Read the model definition and answer for the solid it produces. Units are mm, in the model's axes. A direction names the side the tool comes from. Coordinates: 2 decimals unless noted, no trailing zeros. Loops run counter-clockwise (first coordinate to the right, second up) from the corner with the lowest first, then second, coordinate; pieces in that order, holes last. Notation, with made-up numbers: M -32,-8.75 L 16,-8.75 A20 ccw 16,15.25 Z; hole C 81.25,58.25 d5. An arc over 180 degrees is marked long. One line per item, written item: value. Start each with the question number.
1. Consider probe 1 along Z at (x, y) = (-10, -9.3); probe 2 along Z at (x, y) = (17, 0.25); probe 3 along Y at (x, z) = (26.5, 3.5). Determine where each line is inside the solid, lowest interval first.
2. Flat-ended cylindrical pins translate along their axes: pin 1 (2.5 mm diameter, centred on x = 13, y = 2.5, fed in from +Z); pin 2 (2 mm diameter, centred on y = -2.5, z = 19, fed in from -X); pin 3 (4 mm diameter, centred on y = -5.5, z = 48, fed in from +X). Find the tip coordinate at first contact, or state that the pin passes through.
3. The part is cut by section C-C (y = -8.5). Write down the section's boundary in (x, z).
4. The part is cut by section A-A (x = -10). Write down the section's boundary in (y, z).
5. Determine the mould class of faces 4 (the face through (0, -1, 30)), 5 (the face through (19, -1.95, 4)), 6 (the face through (4, -4.1, 23)) for opening direction Y: +Y half, -Y half, draft (parallel to the pull), parting line (faces both ways), or undercut.
6. For faces 1 (the face through (5.039, -1, 56)), 2 (the face through (-12, -7.081, 3)), 3 (the face through (7, 1, 55)), determine the directions among +Z, -Z, +X, -X, +Y, -Y from which every point of the face is accessible in a straight line to the end or side of a thin tool.
```python
from build123d import *

# Parameters (mm, degrees)
PAD_DEPTH       = 12
SKETCH001_R     = 3
HOLE_DEPTH      = 13.001
PAD001_DEPTH    = 7
SKETCH003_W     = 28
SKETCH003_H     = 2.7
POCKET_DEPTH    = 2
SKETCH004_W     = 4
SKETCH004_H     = 2.7
POCKET001_DEPTH = 2.5


with BuildPart() as part:
    # Sketch → Pad (new body)
    with BuildSketch(Plane.XY):
        Polygon((-20, -10.081048), (5, -10.081048), (5, 2.918952), (0, 2.918952), (0, -7.081048), (-20, -7.081048), align=None)
    extrude(amount=PAD_DEPTH)

    # Sketch001 (on Face1 of Pad) → Hole (cut, through all)
    with BuildSketch(Plane.XZ.offset(10.081048)):
        with Locations((-10, 6)):
            Circle(SKETCH001_R)
    extrude(amount=-HOLE_DEPTH, mode=Mode.SUBTRACT)

    # Sketch002 → Pad001 (join)
    with BuildSketch(Plane.XZ.offset(-2.9)):
        Polygon((33.008904, 5), (33.008904, 0), (0, 0), (0, 11.991246), (0, 60), (9.008904, 60), (9.008904, 55), (5.008904, 55), (5.008904, 5), align=None)
    extrude(amount=PAD001_DEPTH)

    # Sketch003 (on Face15 of Pad001) → Pocket (cut)
    with BuildSketch(Plane(origin=(0, -6, 5), x_dir=(1, 0, 0), z_dir=(0, 0, 1))):
        with Locations((19.008904, 5.4)):
            Rectangle(SKETCH003_W, SKETCH003_H)
    extrude(amount=-POCKET_DEPTH, mode=Mode.SUBTRACT)

    # Sketch004 (on Face17 of Pocket) → Pocket001 (cut)
    with BuildSketch(Plane(origin=(54, 23, 55), x_dir=(1, 0, 0), z_dir=(0, 0, -1))):
        with Locations((-46.961428, 23.6)):
            Rectangle(SKETCH004_W, SKETCH004_H)
    extrude(amount=-POCKET001_DEPTH, mode=Mode.SUBTRACT)


solid = part.part
```
Answer block:
1. probe 1: z = 0 to 3, 9 to 12
1. probe 2: z = 0 to 3
1. probe 3: y = -4.1 to -1.95, 0.75 to 2.9
2. pin 1: stops at z = 5
2. pin 2: stops at x = 0
2. pin 3: stops at x = 5.01
3. outline: M -20,0 L 5,0 L 5,12 L -20,12 Z; hole C -10,6 d6
4. outline: M -10.08,0 L -7.08,0 L -7.08,3 L -10.08,3 Z; M -10.08,9 L -7.08,9 L -7.08,12 L -10.08,12 Z
5. face 4: draft
5. face 5: undercut
5. face 6: -Y half
6. face 1: +X
6. face 2: +Z, -Z, -X, +Y
6. face 3: +X, +Y, -Y
